The model under review builds one solid part; all positions refer to its coordinate system, in mm. A direction names the side the tool comes from. Round coordinates to 2 decimals unless told otherwise and drop trailing zeros. Write each loop counter-clockwise with the first axis right and the second up, starting at its lowest first coordinate (ties: lowest second). Pieces come first, ordered by that corner, then holes. Notation, with made-up numbers: (34, -18) - (73, -18) arc R24 cw to (73, 14) - close; hole circle Ø2 at (51, -32). An arc over 180 degrees is marked (long way). One line per question, with ' | ' between items. Start each with the question number.
```python
from build123d import *

# Parameters (mm, degrees)
SKETCH1_W           = 59
SKETCH1_H           = 27
SKETCH1_R           = 1.5
BOSS_EXTRUDE1_DEPTH = 1
SKETCH2_W           = 34
SKETCH2_H           = 18
BOSS_EXTRUDE2_DEPTH = 7
SKETCH3_W           = 4
SKETCH3_H           = 18
BOSS_EXTRUDE3_DEPTH = 15
SKETCH4_W           = 4
SKETCH4_H           = 18
BOSS_EXTRUDE4_DEPTH = 15
SKETCH7_W           = 10
SKETCH7_H           = 12
BOSS_EXTRUDE7_DEPTH = 5
SKETCH8_W           = 6
SKETCH8_H           = 6.85
BOSS_EXTRUDE8_DEPTH = 1.8


with BuildPart() as part:
    # Sketch1 → Boss-Extrude1 (new body)
    with BuildSketch(Plane(origin=(0, 0, 0), x_dir=(1, 0, 0), z_dir=(0, 1, 0))):
        with Locations((1.308219178, 7.805712308)):
            Rectangle(SKETCH1_W, SKETCH1_H)
        with Locations((-26.191780822, -3.694287692)):
            Circle(SKETCH1_R, mode=Mode.SUBTRACT)
        with Locations((-26.191780822, 19.305712308)):
            Circle(SKETCH1_R, mode=Mode.SUBTRACT)
        with Locations((28.808219178, 19.305712308)):
            Circle(SKETCH1_R, mode=Mode.SUBTRACT)
        with Locations((28.808219178, -3.694287692)):
            Circle(SKETCH1_R, mode=Mode.SUBTRACT)
    extrude(amount=BOSS_EXTRUDE1_DEPTH)

    # Sketch2 → Boss-Extrude2 (add)
    with BuildSketch(Plane(origin=(0, 1, 0), x_dir=(1, 0, 0), z_dir=(0, 1, 0))):
        with Locations((-1.191780822, 6.805712308)):
            Rectangle(SKETCH2_W, SKETCH2_H)
    extrude(amount=BOSS_EXTRUDE2_DEPTH)

    # Sketch3 → Boss-Extrude3 (add)
    with BuildSketch(Plane(origin=(0, 1, 0), x_dir=(1, 0, 0), z_dir=(0, 1, 0))):
        with Locations((-20.191780822, 6.805712308)):
            Rectangle(SKETCH3_W, SKETCH3_H)
    extrude(amount=BOSS_EXTRUDE3_DEPTH)

    # Sketch4 → Boss-Extrude4 (add)
    with BuildSketch(Plane(origin=(0, 1, 0), x_dir=(1, 0, 0), z_dir=(0, 1, 0))):
        with Locations((17.808219178, 6.805712308)):
            Rectangle(SKETCH4_W, SKETCH4_H)
    extrude(amount=BOSS_EXTRUDE4_DEPTH)

    # Sketch7 → Boss-Extrude7 (add)
    with BuildSketch(Plane(origin=(0, 1, 0), x_dir=(1, 0, 0), z_dir=(0, 1, 0))):
        with Locations((25.808219178, 7.805712308)):
            Rectangle(SKETCH7_W, SKETCH7_H)
    extrude(amount=BOSS_EXTRUDE7_DEPTH)

    # Sketch8 → Boss-Extrude8 (add)
    with BuildSketch(Plane(origin=(0, 1, 0), x_dir=(1, 0, 0), z_dir=(0, 1, 0))):
        with Locations((-25.191780822, 7.805712308)):
            Rectangle(SKETCH8_W, SKETCH8_H)
    extrude(amount=BOSS_EXTRUDE8_DEPTH)


solid = part.part
```
1. Machinability: for faces 1 (the face through (26, 6, -8)), 2 (the face through (-25, 2, -11.231)), 3 (the face through (-18.192, 12, -7)), which of the approach directions +Z, -Z, +X, -X, +Y, -Y give a long, thin tool a straight path to every point of the face, cutting with its end or side? Answer none if there is none.
2. Clearance check with flat-ended pins moving along their axes: P1, Ø2, axis at y = 2.5, z = 2, coming from the +X side; P2, Ø4, axis at x = 26, y = 3.5, coming from the +Z side; P3, Ø1, axis at x = -5, z = -0.5, coming from the -Y side; P4, Ø1.5, axis at x = 7.5, y = 2.5, coming from the -Z side. State where each tip first meets the part, or that it passes through.
3. The part is to be moulded in two halves that separate along X. For faces 4 (the face through (30.808, 2, -8)), 5 (the face through (-27.69, 0.49, -19.37)), 6 (the face through (1, 0, -8)), say which applies: pulls with the +X half, pulls with the -X half, needs draft (parallel to the pull), parting line crosses it, or undercut.
4. Add section A-A, the plane y = 3.5. Write out the cut boundary in (x, z).
5. Add section C-C, the plane x = 17. Write out the cut boundary in (y, z), then the cut area to 3 significant figures.
6. Add section D-D, the plane y = 11.25. Write out the cut boundary in (x, z), then the cut area to 3 significant figures.
7. Add section B-B, the plane z = -0.75. Write out the cut boundary in (x, y), then the cut area to 3 significant figures.
8. Wall thickness on line 1 along X through (y, z) = (11, -3.75); line 2 along X through (y, z) = (4.75, -8.75); line 3 along Z through (x, y) = (-7, 6.75): over which ranges is each line inside the solid? List them lowest first. Write a range as [from, to].
Geometry check:
1) face 1: +Z, -Z, +X, +Y | face 2: -Z, -X, +Y | face 3: +Z, -Z, +Y
2) P1: stops at x = 19.81 | P2: stops at z = -1.81 | P3: stops at y = 0 | P4: stops at z = -15.81
3) face 4: pulls with the +X half | face 5: undercut | face 6: needs draft
4) outline: (-22.19, -15.81) - (19.81, -15.81) - (19.81, 2.19) - (-22.19, 2.19) - close; (20.81, -13.81) - (30.81, -13.81) - (30.81, -1.81) - (20.81, -1.81) - close
5) outline: (0, -21.31) - (1, -21.31) - (1, -15.81) - (16, -15.81) - (16, 2.19) - (1, 2.19) - (1, 5.69) - (0, 5.69) - close | area: 297 mm2
6) outline: (-22.19, -15.81) - (-18.19, -15.81) - (-18.19, 2.19) - (-22.19, 2.19) - close; (15.81, -15.81) - (19.81, -15.81) - (19.81, 2.19) - (15.81, 2.19) - close | area: 144 mm2
7) outline: (-28.19, 0) - (30.81, 0) - (30.81, 1) - (19.81, 1) - (19.81, 16) - (15.81, 16) - (15.81, 8) - (-18.19, 8) - (-18.19, 16) - (-22.19, 16) - (-22.19, 1) - (-28.19, 1) - close | area: 417 mm2
8) line 1: x = [-22.19, -18.19], [15.81, 19.81] | line 2: x = [-22.19, 19.81], [20.81, 30.81] | line 3: z = [-15.81, 2.19]
